For this review, use the dimensioned drawing (mm, ordinates from the lowest corner) and the shaded views. A direction names the side the tool comes from. Coordinates: 2 decimals unless noted, no trailing zeros. Order: outer loops, then holes, each group sorted by start corner. A loop starts at its lowest first (then second) coordinate and runs counter-clockwise, first axis right, second up. Notation, with made-up numbers: (5, -6) -> (64, -6) arc R29 cw to (64, 24) -> close; hole circle Ø7 at (46.5, 75). An arc over 180 degrees is marked (long way). Return JSON: item names as keys, results as strings. Group by question number.
Item 1: For line 1 along Y through (x, z) = (1, 3.5); line 2 along Z through (x, y) = (3.5, 4.75); line 3 along X through (y, z) = (13.5, 3), list the stretches that pass through material, from the lowest coordinate up.
Item 2: Take a section at D-D (x = 4). Write out the cut boundary in (y, z), then the cut area to 3 significant figures.
Item 3: Machinability: for the marked faces 1 and 2, which of the approach directions +Z, -Z, +X, -X, +Y, -Y give a long, thin tool a straight path to every point of the face, cutting with its end or side? Answer none if there is none.
Item 4: Insertion check: pin 1 (1.5 mm diameter, centred on y = 23.5, z = 4, fed in from -X); pin 2 (1.5 mm diameter, centred on x = 4, y = 12.5, fed in from +Z). Each pin has a flat end and moves straight along its axis. Give the tip position at first contact, or say it passes through.
Item 5: Take a section at B-B (z = 4). Write out the cut boundary in (x, y).
Item 6: Take a section at C-C (y = 23.5). Write out the cut boundary in (x, z).
Item 7: Take a section at A-A (x = 0.5). Write out the cut boundary in (y, z).
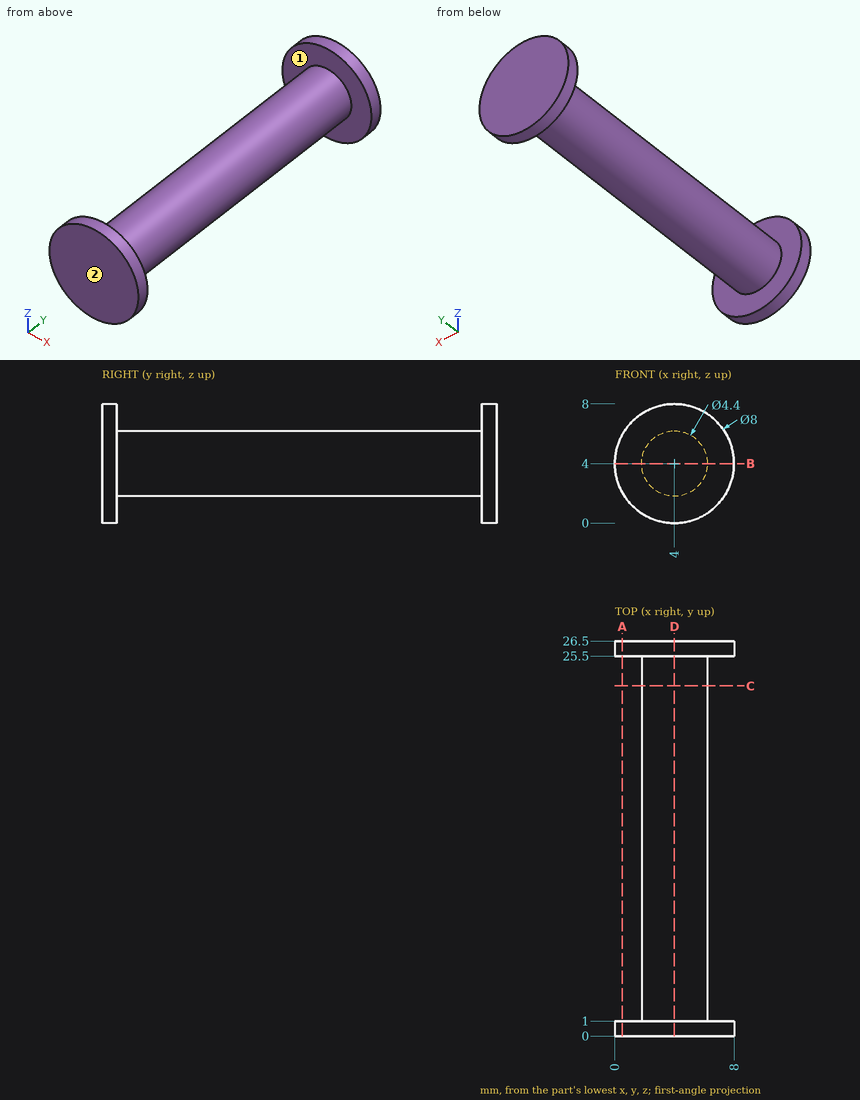
Findings below:
{
 "1": {"line 1": "y = 0 to 1, 25.5 to 26.5", "line 2": "z = 1.86 to 6.14", "line 3": "x = 2.04 to 5.96"},
 "2": {"outline": "(0, 0) -> (1, 0) -> (1, 1.8) -> (25.5, 1.8) -> (25.5, 0) -> (26.5, 0) -> (26.5, 8) -> (25.5, 8) -> (25.5, 6.2) -> (1, 6.2) -> (1, 8) -> (0, 8) -> close", "area": "124 mm2"},
 "3": {"face 1": "none", "face 2": "+Z, -Z, +X, -X, -Y"},
 "4": {"pin 1": "stops at x = 1.8", "pin 2": "stops at z = 6.2"},
 "5": {"outline": "(0, 0) -> (8, 0) -> (8, 1) -> (6.2, 1) -> (6.2, 25.5) -> (8, 25.5) -> (8, 26.5) -> (0, 26.5) -> (0, 25.5) -> (1.8, 25.5) -> (1.8, 1) -> (0, 1) -> close"},
 "6": {"outline": "circle Ø4.4 at (4, 4)"},
 "7": {"outline": "(0, 2.06) -> (1, 2.06) -> (1, 5.94) -> (0, 5.94) -> close; (25.5, 2.06) -> (26.5, 2.06) -> (26.5, 5.94) -> (25.5, 5.94) -> close"}
}
